Part print with two shaded views. Sizes in mm from the minimum x, y, z corner. A direction names the side the tool comes from. Give positions to 0.01 mm unless a question says otherwise; leave off trailing zeros. Write each loop counter-clockwise with the first axis right and the second up, starting at its lowest first coordinate (ties: lowest second). Pieces come first, ordered by that corner, then holes. Notation, with made-up numbers: M 75,23.25 L 129,23.25 A12 ccw 129,43.25 Z; hole C -9.5,52.25 d4. An arc over 180 degrees is marked long. Return JSON: item names as keys, results as strings. Group by question number.
Q1. Flat gauge pins, fed straight in: pin 1 Ø3 at (x, y) = (40, 2.5) entering from +Z (3 decimals); pin 2 Ø1 at (y, z) = (3.5, 5) entering from -X; pin 3 Ø0.6 at (y, z) = (3.5, 5) entering from +X. Where does each tip first touch, or does it go through?
Q2. Tool access for the marked faces 1, 2 and 3: list every direction of +Z, -Z, +X, -X, +Y, -Y with a clear straight run to the whole face (end or side of a thin tool).
Q3. Band-saw the part on A-A, the plane y = 1.75. Give the cut face in (x, z) (3 decimals).
Q4. Band-saw the part on C-C, the plane z = 0.5. Give the cut face in (x, y).
Q5. Band-saw the part on D-D, the plane y = 4. Give the cut face in (x, z) (3 decimals).
Q6. Wall check: probe 1 along X at (y, z) = (3.75, 4.5); probe 2 along Y at (x, z) = (18, 5.5); probe 3 along Z at (x, y) = (42, 2.5) (3 decimals). Give the ranges that are in metal, low to high.
Q7. Band-saw the part on B-B, the plane x = 3.5. Give the cut face in (y, z) (3 decimals), then the cut area to 3 significant figures.
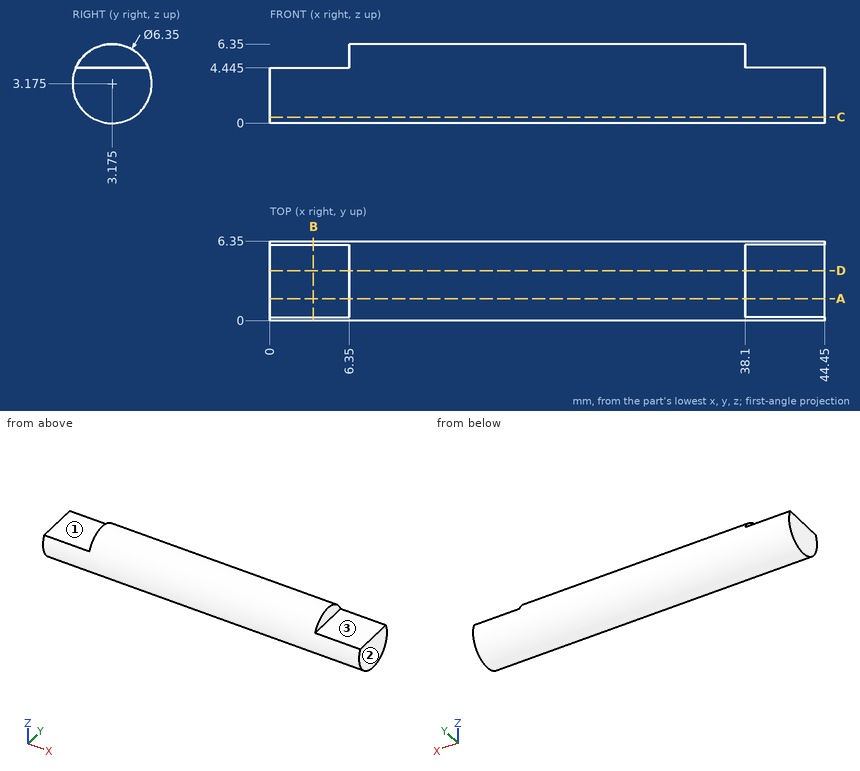
From the geometry:
{
 "1": {"pin 1": "stops at z = 4.445", "pin 2": "stops at x = 6.35", "pin 3": "stops at x = 38.1"},
 "2": {"face 1": "+Z, -X, +Y, -Y", "face 2": "+Z, -Z, +X, +Y, -Y", "face 3": "+Z, +X, +Y, -Y"},
 "3": {"outline": "M 0,0.338 L 44.45,0.338 L 44.45,4.445 L 38.1,4.445 L 38.1,6.012 L 6.35,6.012 L 6.35,4.445 L 0,4.445 Z"},
 "4": {"outline": "M 0,1.46 L 44.45,1.46 L 44.45,4.89 L 0,4.89 Z"},
 "5": {"outline": "M 0,0.109 L 44.45,0.109 L 44.45,4.445 L 38.1,4.445 L 38.1,6.241 L 6.35,6.241 L 6.35,4.445 L 0,4.445 Z"},
 "6": {"probe 1": "x = 6.35 to 38.1", "probe 2": "y = 1.01 to 5.34", "probe 3": "z = 0.073 to 4.445"},
 "7": {"outline": "M 0.265,4.445 A3.175 ccw long 6.085,4.445 Z", "area": "23.7 mm^2"}
}
